```python
from build123d import *

# Parameters (mm, degrees)
BOSS_EXTRUDE1_DEPTH   = 5
SKETCH2_OUTSIDE_W     = 36.254
SKETCH2_OUTSIDE_H     = 34.474
SKETCH2_OUTSIDE_R     = 5.75
CUT_EXTRUDE1_DEPTH    = 5
CUT_EXTRUDE1_DRAFT    = -60
SKETCH3_OUTSIDE_W     = 36.254
SKETCH3_OUTSIDE_H     = 34.474
SKETCH3_OUTSIDE_R     = 5.75
CUT_EXTRUDE2_DEPTH    = 5
CUT_EXTRUDE2_DRAFT    = -60
M6_TAPPED_HOLE1_D     = 5
M6_TAPPED_HOLE1_DEPTH = 17


with BuildPart() as part:
    # Sketch1 → Boss-Extrude1 (new body)
    with BuildSketch(Plane(origin=(0, 0, 0), x_dir=(1, 0, 0), z_dir=(0, 1, 0))):
        Polygon((6.639528096, 0), (3.319764048, 5.75), (-3.319764048, 5.75), (-6.639528096, 0), (-3.319764048, -5.75), (3.319764048, -5.75), align=None)
    extrude(amount=BOSS_EXTRUDE1_DEPTH)


with BuildPart() as cut_extrude1_tool:
    # Sketch2 outside → Cut-Extrude1 (with draft: the straight prism first)
    with BuildSketch(Plane(origin=(0, 5, 0), x_dir=(1, 0, 0), z_dir=(0, 1, 0))):
        Rectangle(SKETCH2_OUTSIDE_W, SKETCH2_OUTSIDE_H)
        Circle(SKETCH2_OUTSIDE_R, mode=Mode.SUBTRACT)
    extrude(amount=-CUT_EXTRUDE1_DEPTH)
    # Cut-Extrude1: the draft: its side faces are tilted about the plane it starts from
    cut_extrude1_sides = [cut_extrude1_tool.faces().sort_by_distance(p)[0] for p in [
        (0, 2.5, 17.237),
        (18.127, 2.5, 0),
        (0, 2.5, -17.237),
        (-18.127, 2.5, 0),
        (-5.75, 2.5, 0),
    ]]
    draft(cut_extrude1_sides, Plane(origin=(0, 5, 0), x_dir=(1, 0, 0), z_dir=(0, 1, 0)), CUT_EXTRUDE1_DRAFT)


with BuildPart() as part_1:
    add(part.part)

    # Cut-Extrude1: cut by cut_extrude1_tool
    add(cut_extrude1_tool.part, mode=Mode.SUBTRACT)


with BuildPart() as cut_extrude2_tool:
    # Sketch3 outside → Cut-Extrude2 (with draft: the straight prism first)
    with BuildSketch(Plane.XZ):
        Rectangle(SKETCH3_OUTSIDE_W, SKETCH3_OUTSIDE_H)
        Circle(SKETCH3_OUTSIDE_R, mode=Mode.SUBTRACT)
    extrude(amount=-CUT_EXTRUDE2_DEPTH)
    # Cut-Extrude2: the draft: its side faces are tilted about the plane it starts from
    cut_extrude2_sides = [cut_extrude2_tool.faces().sort_by_distance(p)[0] for p in [
        (0, 2.5, -17.237),
        (18.127, 2.5, 0),
        (0, 2.5, 17.237),
        (-18.127, 2.5, 0),
        (-5.75, 2.5, 0),
    ]]
    draft(cut_extrude2_sides, Plane.XZ, CUT_EXTRUDE2_DRAFT)


with BuildPart() as part_2:
    add(part_1.part)

    # Cut-Extrude2: cut by cut_extrude2_tool
    add(cut_extrude2_tool.part, mode=Mode.SUBTRACT)

    # M6 Tapped Hole1
    with Locations(Plane(origin=(0, 5, 0), x_dir=(1, 0, 0), z_dir=(0, 1, 0))):
        with Locations((0, 0)):
            Hole(M6_TAPPED_HOLE1_D / 2, depth=M6_TAPPED_HOLE1_DEPTH)


solid = part_2.part
```
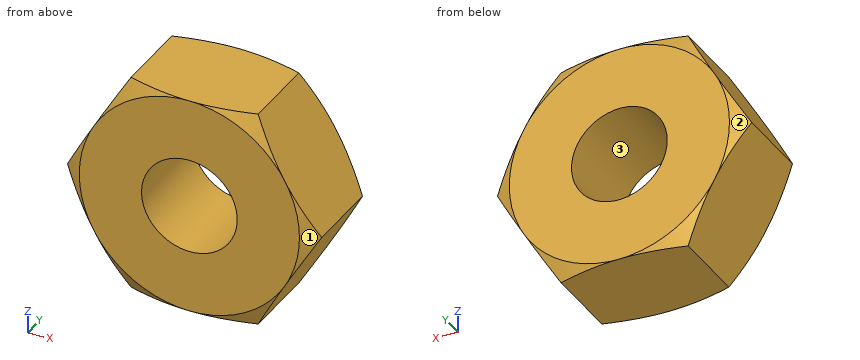
Verification items for the finished model (mm, model axes). Face numbers are marked on the shaded views. Round coordinates to 2 decimals unless told otherwise and drop trailing zeros. Write each loop counter-clockwise with the first axis right and the second up, starting at its lowest first coordinate (ties: lowest second). Pieces come first, ordered by that corner, then holes.
1. Scan lines: L1, parallel to Z at x = 0.5, y = 0.2; L2, parallel to X at y = 4.5, z = -0.25; L3, parallel to X at y = 1.8, z = -3.75. Record each from-to range of solid material in increasing order.
2. Section check A-A on y = 1. Enter the section's corners in (x, z), plus the area to 3 significant figures.
3. Draft check along X on the marked faces 1, 2 and 3. Enter one of: +X half, -X half, draft (parallel to the pull), parting line (faces both ways), or undercut.
Answer:
1. L1: z = -5.75 to -2.45, 2.45 to 5.75
1. L2: x = -6.5 to -2.49, 2.49 to 6.5
1. L3: x = -4.47 to 4.47
2. outline: (-6.64, 0) - (-3.32, -5.75) - (3.32, -5.75) - (6.64, 0) - (3.32, 5.75) - (-3.32, 5.75) - close; hole circle Ø5 at (0, 0)
2. area: 94.9 mm2
3. face 1: +X half
3. face 2: -X half
3. face 3: undercut
